Can you work these out from the model? Positions are in its coordinate system, mm. A direction names the side the tool comes from. Round coordinates to 2 decimals unless told otherwise and drop trailing zeros. Order: outer loops, then holes, each group sorted by start corner. A loop starts at its lowest first (then second) coordinate and runs counter-clockwise, first axis right, second up. Notation, with made-up numbers: (25, 65) -> (65, 65) arc R19 ccw to (65, 97) -> close; hole circle Ø2 at (0.5, 72). An arc over 180 degrees is marked (long way). Use a Markdown table: item, result. Add a question column.
Q1. I'm going to push flat-ended pins straight in: pin 1 Ø12.5 at (x, z) = (-7, 15.5) entering from +Y; pin 2 Ø2.5 at (y, z) = (25.5, 6.5) entering from +X; pin 3 Ø1.9 at (x, z) = (14.69, 20.14) entering from -Y. Where does each tip first touch, or does it pass through?
Q2. If we section it at B-B on x = 18: List the corners of the cut face in (y, z) for me, plus the area to 3 significant figures.
Q3. I need wall thicknesses on line 1 along Y through (x, z) = (-22.5, 11.5); line 2 along Y through (x, z) = (-14, 17); line 3 along X through (y, z) = (17.5, 22.5). Which ranges of each line are inside material? Lowest first, please. Write a range as [from, to].
Q4. If we section it at C-C on z = 2.25: List the corners of the cut face in (x, y) for me (3 decimals).
Q5. If we section it at D-D on y = -12.5: List the corners of the cut face in (x, z) for me, plus the area to 3 significant figures.
Q6. For faces 1 (the face through (-17.059, 25, 13)), 2 (the face through (-20, 23.812, 13)), 3 (the face through (-3, -23.813, 13)), 4 (the face through (-20.173, 25.377, 7.865)), which set-ups out of +Z, -Z, +X, -X, +Y, -Y let a thin tool reach every point of the face, with its end or its side?
Q7. If we section it at A-A on z = 12.7: List the corners of the cut face in (x, y) for me (3 decimals), plus the area to 3 significant figures.
Q8. We'd pull the mould along Z, two halves only. Please class faces 5 (the face through (15.887, -22.248, 20.299)), 6 (the face through (-25.68, -19.68, 12.88)), 7 (the face through (-27, -6, 25.4)), 8 (the face through (-27, -6, 0)): +Z half, -Z half, draft (parallel to the pull), parting line (faces both ways), or undercut.
```python
from build123d import *

# Parameters (mm, degrees)
BOSS_EXTRUDE1_DEPTH       = 25.4
M4X0_7_TAPPED_HOLE1_D     = 3.3
M4X0_7_TAPPED_HOLE1_DEPTH = 9.906
M4X0_7_TAPPED_HOLE1_TIP   = 0.991420021
CUT_EXTRUDE1_REACH        = 66.12
SKETCH7_R                 = 5.08
SKETCH7_R_2               = 1.2065
FILLET1_R                 = 3.175
FILLET2_R                 = 3.175


with BuildPart() as part:
    # Sketch1 → Boss-Extrude1 (new body)
    with BuildSketch(Plane.XY):
        Polygon((-17.059275079, 26.987213855), (-29.759275079, 26.987213855), (-29.759275079, -23.812786145), (21.040724921, -23.812786145), (21.040724921, -20.637786145), (-26.584275079, -20.637786145), (-26.584275079, 23.812213855), (-17.059275079, 23.812213855), align=None)
    extrude(amount=BOSS_EXTRUDE1_DEPTH)

    # M4x0.7 Tapped Hole1
    with Locations(Plane(origin=(0, 26.987213855, 0), x_dir=(1, 0, 0), z_dir=(0, 1, 0))):
        with Locations((-21.821775079, -7.9375), (-21.821775079, -17.4625)):
            Hole(M4X0_7_TAPPED_HOLE1_D / 2, depth=M4X0_7_TAPPED_HOLE1_DEPTH)
            with Locations((0, 0, -(M4X0_7_TAPPED_HOLE1_DEPTH + M4X0_7_TAPPED_HOLE1_TIP / 2))):  # 118° drill point
                Cone(0, M4X0_7_TAPPED_HOLE1_D / 2, M4X0_7_TAPPED_HOLE1_TIP, mode=Mode.SUBTRACT)

    # Sketch7 → Cut-Extrude1 (cut, up to next)
    with BuildSketch(Plane.XZ.offset(23.812786145), mode=Mode.PRIVATE) as cut_extrude1_sk1:
        with Locations(Location((14.690724921, 12.7, 0), (0, 0, 270))):
            Circle(SKETCH7_R)
    cut_extrude1_tool1 = extrude(cut_extrude1_sk1.sketch, amount=-CUT_EXTRUDE1_REACH, mode=Mode.PRIVATE) & part.part
    # Sketch7 → Cut-Extrude1 (cut, up to next)
    with BuildSketch(Plane.XZ.offset(23.812786145), mode=Mode.PRIVATE) as cut_extrude1_sk2:
        with Locations(Location((14.690724921, 5.2578, 0), (0, 0, 270))):
            Circle(SKETCH7_R_2)
    cut_extrude1_tool2 = extrude(cut_extrude1_sk2.sketch, amount=-CUT_EXTRUDE1_REACH, mode=Mode.PRIVATE) & part.part
    # Sketch7 → Cut-Extrude1 (cut, up to next)
    with BuildSketch(Plane.XZ.offset(23.812786145), mode=Mode.PRIVATE) as cut_extrude1_sk3:
        with Locations(Location((14.690724921, 20.1422, 0), (0, 0, 270))):
            Circle(SKETCH7_R_2)
    cut_extrude1_tool3 = extrude(cut_extrude1_sk3.sketch, amount=-CUT_EXTRUDE1_REACH, mode=Mode.PRIVATE) & part.part
    add(cut_extrude1_tool1.solids().sort_by_distance((14.690725, -23.812786, 12.7))[0], mode=Mode.SUBTRACT)
    add(cut_extrude1_tool2.solids().sort_by_distance((14.690725, -23.812786, 5.2578))[0], mode=Mode.SUBTRACT)
    add(cut_extrude1_tool3.solids().sort_by_distance((14.690725, -23.812786, 20.1422))[0], mode=Mode.SUBTRACT)

    # Fillet1
    fillet1_edges = [part.edges().sort_by_distance(p)[0] for p in [
        (-29.759275079, -23.812786145, 12.7),
        (-29.759275079, 26.987213855, 12.7),
    ]]
    fillet(fillet1_edges, radius=FILLET1_R)

    # Fillet2
    fillet2_edges = [part.edges().sort_by_distance(p)[0] for p in [
        (-26.584275079, 23.812213855, 12.7),
        (-26.584275079, -20.637786145, 12.7),
    ]]
    fillet(fillet2_edges, radius=FILLET2_R)


solid = part.part
```
Answer below:
| question | item | result |
|---|---|---|
| 1 | pin 1 | y = -20.64 |
| 1 | pin 2 | x = -17.06 |
| 1 | pin 3 | through |
| 2 | outline | (-23.81, 0) -> (-20.64, 0) -> (-20.64, 8.85) -> (-23.81, 8.85) -> close; (-23.81, 16.55) -> (-20.64, 16.55) -> (-20.64, 25.4) -> (-23.81, 25.4) -> close |
| 2 | area | 56.2 mm² |
| 3 | line 1 | [-23.81, -20.64], [23.81, 26.99] |
| 3 | line 2 | [-23.81, -20.64] |
| 3 | line 3 | [-29.76, -26.58] |
| 4 | outline | (-29.759, -20.638) arc R3.175 ccw to (-26.584, -23.813) -> (21.041, -23.813) -> (21.041, -20.638) -> (-23.409, -20.638) arc R3.175 cw to (-26.584, -17.463) -> (-26.584, 20.637) arc R3.175 cw to (-23.409, 23.812) -> (-17.059, 23.812) -> (-17.059, 26.987) -> (-26.584, 26.987) arc R3.175 ccw to (-29.759, 23.812) -> close |
| 5 | outline | (-29.76, 0) -> (-26.58, 0) -> (-26.58, 25.4) -> (-29.76, 25.4) -> close |
| 5 | area | 80.6 mm² |
| 6 | face 1 | +Z, -Z, +X, +Y |
| 6 | face 2 | +Z, -Z, +X |
| 6 | face 3 | +Z, -Z, +X, -X, -Y |
| 6 | face 4 | +Y |
| 7 | outline | (-29.759, -20.638) arc R3.175 ccw to (-26.584, -23.813) -> (9.611, -23.813) -> (9.611, -20.638) -> (-23.409, -20.638) arc R3.175 cw to (-26.584, -17.463) -> (-26.584, 20.637) arc R3.175 cw to (-23.409, 23.812) -> (-17.059, 23.812) -> (-17.059, 26.987) -> (-26.584, 26.987) arc R3.175 ccw to (-29.759, 23.812) -> close; (19.771, -23.813) -> (21.041, -23.813) -> (21.041, -20.638) -> (19.771, -20.638) -> close |
| 7 | area | 310 mm² |
| 8 | face 5 | undercut |
| 8 | face 6 | draft |
| 8 | face 7 | +Z half |
| 8 | face 8 | -Z half |
